Here's how the part is built. I have some questions about the finished solid (model axes, mm). A direction names the side the tool comes from. Coordinates: 2 decimals unless noted, no trailing zeros. Write each loop counter-clockwise with the first axis right and the second up, starting at its lowest first coordinate (ties: lowest second). Pieces come first, ordered by that corner, then holes.
(1) Imagine slicing it at C-C, the plane z = 27. List the corners of the cut face in (x, y) for me, plus the area to 3 significant figures.
(2) Thinking about a two-plate mould opening in X: for faces 1 (the flat face through (-31.776, -10, 5)), 2 (the cylindrical face through (-7.32, -9.86, 7.53)), 3 (the cylindrical face through (-34.98, -10.13, 6.23)), 4 (the cylindrical face through (-33.04, -0.3, 6.23)), which applies, released by +X, released by -X, zero draft, split by the parting line, or undercut?
(3) For pin 1 Ø10.5 at (y, z) = (-5, 26.5) entering from -X; pin 2 Ø2.5 at (y, z) = (-14, 25.5) entering from +X; pin 3 Ø6 at (x, y) = (7, -12) entering from +Z; pin 4 Ø1 at (x, z) = (-8, 9.5) entering from -Y, each with a flat end and sliding along its axis, tell me the tip position at first contact or that it passes through.
(4) Which directions (+Z, -Z, +X, -X, +Y, -Y) give clear straight access to the entire face, cutting with the end or side of a thin tool? Please do faces 5 (the cylindrical face through (-9.245, -0.301, 22.276)), 6 (the flat face through (-24, -10, 3.518)), 7 (the flat face through (-33, -10, 6.518)).
(5) Imagine slicing it at A-A, the plane y = -18. List the corners of the cut face in (x, z) for me, plus the area to 3 significant figures.
(6) Imagine slicing it at D-D, the plane x = -29.5. List the corners of the cut face in (y, z) for me.
(7) Imagine slicing it at B-B, the plane x = 12. List the corners of the cut face in (y, z) for me, plus the area to 3 significant figures.
(8) Please list where these lines run through material, in increasing order: probe 1 along X at (y, z) = (-18.25, 26); probe 2 along Z at (x, y) = (8, -10); probe 3 along Z at (x, y) = (-25, -5.5).
```python
from build123d import *

# Parameters (mm, degrees)
F1_DEPTH = 20
F2_DEPTH = 20
F3_W     = 20
F3_H     = 20
F4_DEPTH = 15
F5_R     = 5.1
F6_DEPTH = 15
F7_R     = 1


# Not quite as in the source:
# - a feature names something its author has since deleted; it is built from what else it names


with BuildPart() as f1:
    # F0 (on Front) → F1 (new body)
    with BuildSketch(Plane.XZ):
        with BuildLine():
            Line((-11.0182737141, 21.9913642435), (-7.5182737801, 21.9906845019))
            Line((-7.5182737801, 21.9906845019), (-7.5182737801, 29.8039734362))
            Line((-7.5182737801, 29.8039734362), (-3.5182737801, 29.8039734362))
            Line((-3.5182737801, 29.8039734362), (-3.5182737801, 16.8525947745))
            ThreePointArc((-3.5182737801, 16.8525947745), (-7.4238059768, 7.4238059768), (-16.8525947745, 3.5182737801))
            Line((-16.8525947745, 3.5182737801), (-31.7764421987, 3.5182737801))
            Line((-31.7764421987, 3.5182737801), (-31.7764421987, 6.5182737801))
            Line((-31.7764421987, 6.5182737801), (-35.2764421987, 6.5182737801))
            Line((-35.2764421987, 6.5182737801), (-35.2764421987, 0))
            Line((-35.2764421987, 0), (-16.8525947745, 0))
            ThreePointArc((-16.8525947745, 0), (-4.9360107289, 4.9360107289), (0, 16.8525947745))
            Line((0, 16.8525947745), (0, 29.8039734362))
            ThreePointArc((0, 29.8039734362), (-1.0304785321, 32.2917686842), (-3.5182737801, 33.3222472163))
            Line((-3.5182737801, 33.3222472163), (-7.5182737801, 33.3222472163))
            ThreePointArc((-7.5182737801, 33.3222472163), (-10.0040648606, 32.2914241533), (-11.0308766315, 29.8039734362))
            Line((-11.0308766315, 29.8039734362), (-11.0182737141, 21.9913642435))
        make_face()
    extrude(amount=F1_DEPTH)

    # F0 (on Front) → F2 (join)
    with BuildSketch(Plane.XZ):
        with BuildLine():
            Line((0, 0), (0, 16.8525947745))
            ThreePointArc((0, 16.8525947745), (-4.9360107289, 4.9360107289), (-16.8525947745, 0))
            Line((-16.8525947745, 0), (0, 0))
        make_face()
    extrude(amount=F2_DEPTH)

    # F3 (on face) → F4 (join)
    with BuildSketch(Plane.YZ):
        with Locations((-10, 10)):
            Rectangle(F3_W, F3_H)
    extrude(amount=F4_DEPTH)

    # F5 (on face) → F6 (cut)
    with BuildSketch(Plane.YZ.offset(15)):
        with Locations((-10, 10)):
            Circle(F5_R)
    extrude(amount=-F6_DEPTH, mode=Mode.SUBTRACT)

    # F7
    f7_edges = [f1.edges().sort_by_distance(p)[0] for p in [
        (-10.138221, -20, 0),
        (-10.138221, 0, 0),
        (-35.276442, -10, 0),
        (-35.276442, -10, 6.518274),
        (-35.276442, 0, 3.259137),
        (-35.276442, -20, 3.259137),
        (-33.526442, -20, 6.518274),
        (-33.526442, 0, 6.518274),
        (-9.268274, 0, 21.991024),
        (-9.268274, -20, 21.991024),
        (-11.018274, -10, 21.991364),
        (7.5, 0, 20),
        (7.5, -20, 20),
        (15, 0, 10),
        (15, -10, 20),
        (15, -20, 10),
        (15, -10, 0),
    ]]
    fillet(f7_edges, radius=F7_R)


solid = f1.part
```
Recorded:
1. outline: (-11.03, -20) - (-7.52, -20) - (-7.52, 0) - (-11.03, 0) - close; (-3.52, -20) - (0, -20) - (0, 0) - (-3.52, 0) - close
1. area: 141 mm2
2. face 1: undercut
2. face 2: undercut
2. face 3: released by -X
2. face 4: zero draft
3. pin 1: stops at x = -11.03
3. pin 2: stops at x = 0
3. pin 3: stops at z = 20
3. pin 4: passes through
4. face 5: -X, +Y
4. face 6: +Z, +Y, -Y
4. face 7: +Z, -X, +Y, -Y
5. outline: (-35.28, 1) arc R1 ccw to (-34.28, 0) - (14, 0) arc R1 ccw to (15, 1) - (15, 19) arc R1 ccw to (14, 20) - (0, 20) - (0, 29.8) arc R3.52 ccw to (-3.52, 33.32) - (-7.52, 33.32) arc R3.51 ccw to (-11.03, 29.8) - (-11.02, 22.99) arc R1 ccw to (-10.02, 21.99) - (-7.52, 21.99) - (-7.52, 29.8) - (-3.52, 29.8) - (-3.52, 16.85) arc R13.33 cw to (-16.85, 3.52) - (-31.78, 3.52) - (-31.78, 6.52) - (-34.28, 6.52) arc R1 ccw to (-35.28, 5.52) - close
5. area: 625 mm2
6. outline: (-20, 1) arc R1 ccw to (-19, 0) - (-1, 0) arc R1 ccw to (0, 1) - (0, 3.52) - (-20, 3.52) - close
7. outline: (-20, 1) arc R1 ccw to (-19, 0) - (-1, 0) arc R1 ccw to (0, 1) - (0, 19) arc R1 ccw to (-1, 20) - (-19, 20) arc R1 ccw to (-20, 19) - close; hole circle Ø10.2 at (-10, 10)
7. area: 317 mm2
8. probe 1: x = -11.02 to -7.52, -3.52 to 0
8. probe 2: z = 0 to 4.9, 15.1 to 20
8. probe 3: z = 0 to 3.52
